from build123d import *

# Parameters (mm, degrees)
SKETCH_R      = 3.11
SKETCH_W      = 12
SKETCH_H      = 8
EXTRUDE_DEPTH = 6


with BuildPart() as part:
    # Sketch → Extrude (new body)
    with BuildSketch(Plane.XY):
        Polygon((0, 0), (135, 0), (135, 140), (90, 190), (45, 190), (0, 140), align=None)
        with Locations((51.3, 146.95)):
            Circle(SKETCH_R, mode=Mode.SUBTRACT)
        with Locations((83.7, 146.95)):
            Circle(SKETCH_R, mode=Mode.SUBTRACT)
        with Locations((51.3, 170.1)):
            Circle(SKETCH_R, mode=Mode.SUBTRACT)
        with Locations((83.7, 170.1)):
            Circle(SKETCH_R, mode=Mode.SUBTRACT)
        with Locations((124, 120.7)):
            Rectangle(SKETCH_W, SKETCH_H, mode=Mode.SUBTRACT)
        with Locations((10, 120.7)):
            Rectangle(SKETCH_W, SKETCH_H, mode=Mode.SUBTRACT)
    extrude(amount=EXTRUDE_DEPTH)


solid = part.part
Model file for the job. Use its own axes, mm. A direction names the side the tool comes from. Coordinates: 2 decimals unless noted, no trailing zeros. Order: outer loops, then holes, each group sorted by start corner. A loop starts at its lowest first (then second) coordinate and runs counter-clockwise, first axis right, second up. Notation, with made-up numbers: M -13,78 L 24,78 A30 cw 24,105 Z; hole C 2,-8 d6. An arc over 180 degrees is marked long. Return JSON: item names as keys, results as strings.
1. Flat gauge pins, fed straight in: pin 1 (1.8 mm diameter, centred on x = 126, z = 4.5, fed in from +Y); pin 2 (3 mm diameter, centred on x = 12, z = 3, fed in from +Y); pin 3 (1 mm diameter, centred on y = 154.5, z = 3, fed in from -X); pin 4 (5.5 mm diameter, centred on x = 51.3, y = 170.1, fed in from +Z). Where does each tip first touch, or does it go through?
Ans:
{"pin 1": "y = 151", "pin 2": "y = 155", "pin 3": "x = 12.6", "pin 4": "through"}
2. Drill centre lines: probe 1 along Y at (x, z) = (83.7, 2.05); probe 2 along X at (y, z) = (146.95, 3.7) (3 decimals); probe 3 along Y at (x, z) = (118.5, 5.65). Where is each one in solid material? Low to high.
Ans:
{"probe 1": "0 to 143.84, 150.06 to 166.99, 173.21 to 190", "probe 2": "6.255 to 48.19, 54.41 to 80.59, 86.81 to 128.745", "probe 3": "0 to 116.7, 124.7 to 158.33"}
3. Tool access for faces 1 (the face through (4, 121, 3)), 2 (the face through (22.815, 165.35, 2.958)): list every direction of +Z, -Z, +X, -X, +Y, -Y with a clear straight run to the whole face (end or side of a thin tool).
Ans:
{"face 1": "+Z, -Z", "face 2": "+Z, -Z, -X, +Y"}
4. Pull direction Y, two halves, no side cores. Call faces 3 (the face through (68, 190, 3)), 4 (the face through (67, 0, 3)), 5 (the face through (10, 116.7, 3)): +Y half, -Y half, draft (parallel to the pull), parting line (faces both ways), or undercut.
Ans:
{"face 3": "+Y half", "face 4": "-Y half", "face 5": "undercut"}
5. Saw through at D-D (x = 14). Give the cut face in (y, z).
Ans:
{"outline": "M 0,0 L 116.7,0 L 116.7,6 L 0,6 Z; M 124.7,0 L 155.56,0 L 155.56,6 L 124.7,6 Z"}
6. Saw through at B-B (z = 3.2). Give the cut face in (x, y).
Ans:
{"outline": "M 0,0 L 135,0 L 135,140 L 90,190 L 45,190 L 0,140 Z; hole M 4,116.7 L 16,116.7 L 16,124.7 L 4,124.7 Z; hole C 51.3,146.95 d6.22; hole C 51.3,170.1 d6.22; hole C 83.7,146.95 d6.22; hole C 83.7,170.1 d6.22; hole M 118,116.7 L 130,116.7 L 130,124.7 L 118,124.7 Z"}
7. Saw through at A-A (x = 83.7). Give the cut face in (y, z).
Ans:
{"outline": "M 0,0 L 143.84,0 L 143.84,6 L 0,6 Z; M 150.06,0 L 166.99,0 L 166.99,6 L 150.06,6 Z; M 173.21,0 L 190,0 L 190,6 L 173.21,6 Z"}
8. Saw through at C-C (y = 170.1). Give the cut face in (x, z), and give its area (3 significant figures).
Ans:
{"outline": "M 27.09,0 L 48.19,0 L 48.19,6 L 27.09,6 Z; M 54.41,0 L 80.59,0 L 80.59,6 L 54.41,6 Z; M 86.81,0 L 107.91,0 L 107.91,6 L 86.81,6 Z", "area": "410 mm^2"}
